Here's the drawing with two shaded views (mm, measured from the low corner). I have some questions. A direction names the side the tool comes from. Give positions to 0.01 mm unless a question says otherwise; leave off trailing zeros. Loops run counter-clockwise (first coordinate to the right, second up) from the corner with the lowest first, then second, coordinate; pieces in that order, holes last. Notation, with made-up numbers: M -35,-31.5 L -8,-31.5 A26 ccw -8,-6.5 Z; hole C -33.75,-15 d11. An arc over 180 degrees is marked long. Put each result on its own line as item: value. Start each with the question number.
1) Imagine slicing it at A-A (y = 5.5). Write out the boundary of the cut face in (x, z), then the cut area to 3 significant figures.
2) For the marked faces 1, 2 and 3, which set-ups out of +Z, -Z, +X, -X, +Y, -Y let a thin tool reach every point of the face, with its end or its side?
3) Imagine slicing it at B-B (z = 12). Write out the boundary of the cut face in (x, y), then the cut area to 3 significant figures.
4) For P1, Ø16, axis at x = 24.5, y = 33, coming from the +Z side, with a flat end and sliding along its axis, tell me the tip position at first contact or that it passes through.
5) If we mould it in two halves opening along X, with no side actions, what happens to the marked faces 4, 5 and 6? For each: +X half, -X half, draft (parallel to the pull), parting line (faces both ways), or undercut.
6) Please list where these lines run through material, in increasing order: line 1 along X through (y, z) = (17.5, 16); line 2 along X through (y, z) = (30, 37.5); line 3 along Z through (x, y) = (20.5, 37.5). Write a range as from..to.
7) Imagine slicing it at C-C (x = 50). Write out the boundary of the cut face in (y, z).
8) Imagine slicing it at D-D (y = 12). Write out the boundary of the cut face in (x, z).
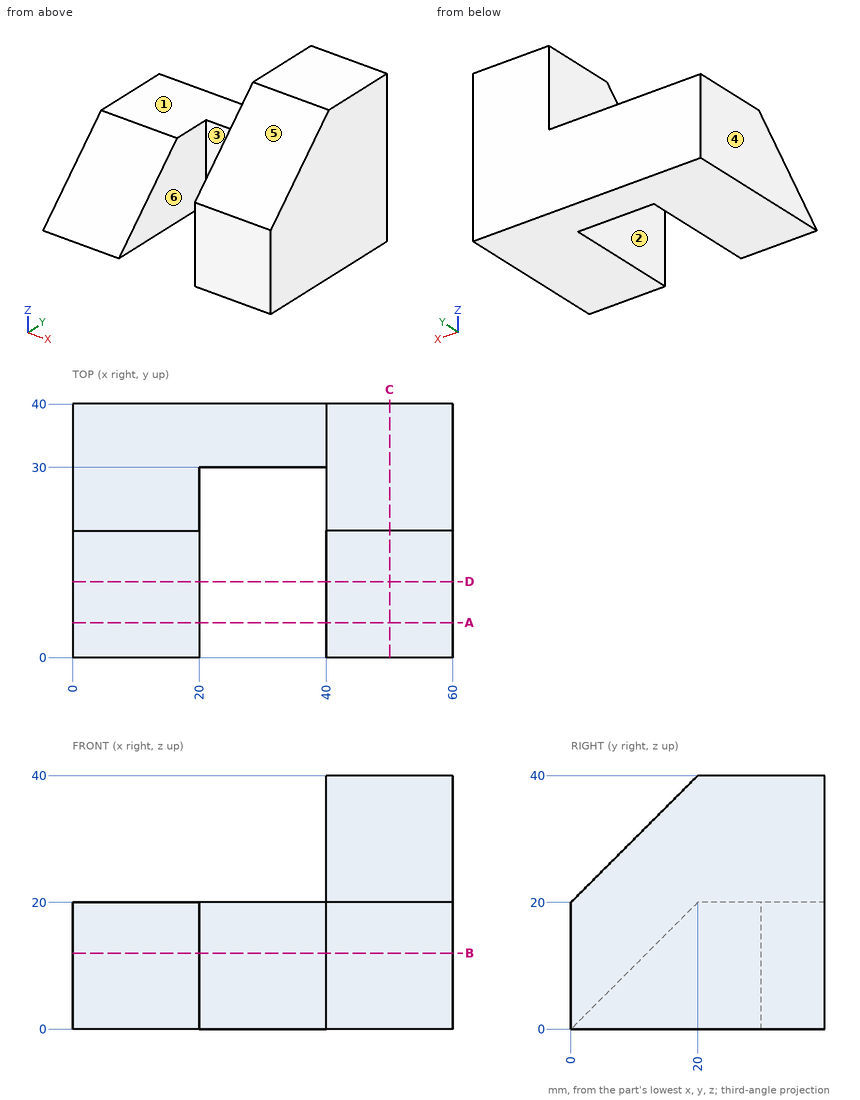
Recorded:
1. outline: M 0,0 L 20,0 L 20,5.5 L 0,5.5 Z; M 40,0 L 60,0 L 60,25.5 L 40,25.5 Z
1. area: 620 mm²
2. face 1: +Z, -X, +Y, -Y
2. face 2: +Z, -Y
2. face 3: +Z, -Z, -Y
3. outline: M 0,12 L 20,12 L 20,30 L 40,30 L 40,0 L 60,0 L 60,40 L 0,40 Z
3. area: 1,560 mm²
4. P1: z = 20
5. face 4: -X half
5. face 5: draft
5. face 6: undercut
6. line 1: 0..20, 40..60
6. line 2: 40..60
6. line 3: 0..20
7. outline: M 0,0 L 40,0 L 40,40 L 20,40 L 0,20 Z
8. outline: M 0,0 L 20,0 L 20,12 L 0,12 Z; M 40,0 L 60,0 L 60,32 L 40,32 Z
